```python
from build123d import *

# Parameters (mm, degrees)
F1_DEPTH = 63.5
F3_DEPTH = 44.45
F5_DEPTH = 18.796


with BuildPart() as f1:
    # F0 (on Top) → F1 (new body)
    with BuildSketch(Plane.XY):
        Polygon((-12.0983748909, -20.955), (12.0983748909, -20.955), (24.1967497817, 0), (12.0983748909, 20.955), (-12.0983748909, 20.955), (-24.1967497817, 0), align=None)
    extrude(amount=F1_DEPTH)

    # F2 (on face) → F3 (cut)
    with BuildSketch(Plane.XY.offset(63.5)):
        Polygon((-11.365140049, -19.685), (11.365140049, -19.685), (22.730280098, 0), (11.365140049, 19.685), (-11.365140049, 19.685), (-22.730280098, 0), align=None)
    extrude(amount=-F3_DEPTH, mode=Mode.SUBTRACT)

    # F4 (on face) → F5 (join)
    with BuildSketch(Plane(origin=(0, 0, 0), x_dir=(1, 0, 0), z_dir=(0, 0, -1))):
        Polygon((-2.286, 20.955), (0, 20.955), (2.286, 20.955), (3.429, 23.241), (0, 23.241), (-3.429, 23.241), align=None)
        Polygon((-20.1272964094, 11.6205), (-18.1475623363, 10.4775), (-17.0045623363, 12.4572340731), (-18.4127964094, 14.5901011096), align=None)
        Polygon((-19.2905623363, 8.4977659269), (-18.1475623363, 10.4775), (-20.1272964094, 11.6205), (-21.8417964094, 8.6508988904), align=None)
        Polygon((-17.0045623363, -12.4572340731), (-18.1475623363, -10.4775), (-20.1272964094, -11.6205), (-18.4127964094, -14.5901011096), align=None)
        Polygon((-20.1272964094, -11.6205), (-18.1475623363, -10.4775), (-19.2905623363, -8.4977659269), (-21.8417964094, -8.6508988904), align=None)
        Polygon((0, -23.241), (0, -20.955), (-2.286, -20.955), (-3.429, -23.241), align=None)
        Polygon((2.286, -20.955), (0, -20.955), (0, -23.241), (3.429, -23.241), align=None)
        Polygon((19.2905623363, -8.4977659269), (18.1475623363, -10.4775), (17.0045623363, -12.4572340731), (18.4127964094, -14.5901011096), (20.1272964094, -11.6205), (21.8417964094, -8.6508988904), align=None)
        Polygon((17.0045623363, 12.4572340731), (18.1475623363, 10.4775), (19.2905623363, 8.4977659269), (21.8417964094, 8.6508988904), (20.1272964094, 11.6205), (18.4127964094, 14.5901011096), align=None)
    extrude(amount=-F5_DEPTH)


solid = f1.part
```
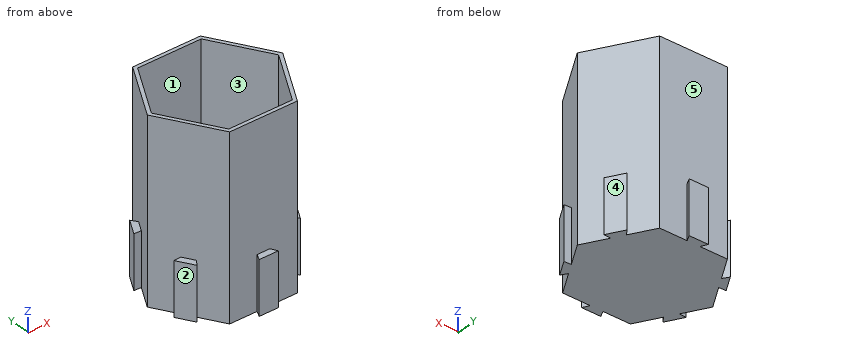
For this review, take the finished solid that the model builds, in its own axes (mm). Face numbers are marked on the shaded views. A direction names the side the tool comes from. Round coordinates to 2 decimals unless told otherwise and drop trailing zeros. Write each loop counter-clockwise with the first axis right and the second up, starting at its lowest first coordinate (ties: lowest second). Pieces come first, ordered by that corner, then holes.
1) Take a section at A-A on x = 21. Give the boundary of the cut face in (y, z), then the cut area to 3 significant figures.
Answer below:
outline: (-10.11, 0) - (-8.6, 0) - (-8.6, 18.8) - (-10.11, 18.8) - close; (-5.54, 0) - (5.54, 0) - (5.54, 63.5) - (3, 63.5) - (3, 19.05) - (-3, 19.05) - (-3, 63.5) - (-5.54, 63.5) - close; (8.6, 0) - (10.11, 0) - (10.11, 18.8) - (8.6, 18.8) - close
area: 493 mm2
2) Insertion check: pin 1 Ø5 at (x, y) = (5, -10) entering from +Z; pin 2 Ø1.5 at (x, z) = (13.5, 20) entering from +Y; pin 3 Ø11.5 at (x, z) = (0.5, 31) entering from +Y (3 decimals). Each pin has a flat end and moves straight along its axis. Give the tip position at first contact, or say it passes through.
Answer below:
pin 1: stops at z = 19.05
pin 2: stops at y = 19.83
pin 3: stops at y = 20.955
3) For line 1 along Y through (x, z) = (-2, 53) (3 decimals); line 2 along X through (y, z) = (-14, 11); line 3 along Z through (x, y) = (-14, 3.5), list the stretches that pass through material, from the lowest coordinate up.
Answer below:
line 1: y = -20.955 to -19.685, 19.685 to 20.955
line 2: x = -18.75 to -18.02, -16.11 to 16.11, 18.02 to 18.75
line 3: z = 0 to 19.05
4) Take a section at C-C on x = 5.5. Give the boundary of the cut face in (y, z) (3 decimals), then the cut area to 3 significant figures.
Answer below:
outline: (-20.955, 0) - (20.955, 0) - (20.955, 63.5) - (19.685, 63.5) - (19.685, 19.05) - (-19.685, 19.05) - (-19.685, 63.5) - (-20.955, 63.5) - close
area: 911 mm2
5) Take a section at B-B on z = 46.5. Give the boundary of the cut face in (x, y) (3 decimals), then the cut area to 3 significant figures.
Answer below:
outline: (-24.197, 0) - (-12.098, -20.955) - (12.098, -20.955) - (24.197, 0) - (12.098, 20.955) - (-12.098, 20.955) - close; hole (-22.73, 0) - (-11.365, -19.685) - (11.365, -19.685) - (22.73, 0) - (11.365, 19.685) - (-11.365, 19.685) - close
area: 179 mm2
6) Mouldability with a two-part tool opening along X and no side actions: class the marked faces 3, 4 and 5 as +X half, -X half, draft (parallel to the pull), parting line (faces both ways), or undercut.
Answer below:
face 3: undercut
face 4: +X half
face 5: draft
7) Machinability: for the marked faces 1 and 2, which of the approach directions +Z, -Z, +X, -X, +Y, -Y give a long, thin tool a straight path to every point of the face, cutting with its end or side? Answer none if there is none.
Answer below:
face 1: +Z
face 2: +Z, -Z, -X, -Y
